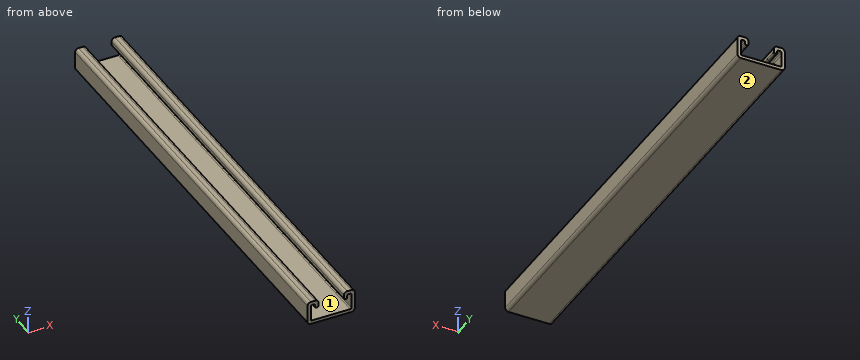
```python
from build123d import *

# Parameters (mm, degrees)
F1_DEPTH = 398
F2_R     = 3
F3_R     = 1


with BuildPart() as f1:
    # F0 (on Front) → F1 (new body)
    with BuildSketch(Plane.XZ):
        Polygon((0, 21), (0, 0), (42, 0), (42, 21), (32.25, 21), (32.25, 14), (35.25, 14), (35.25, 17.75), (39, 17.75), (39, 14), (39, 3), (3, 3), (3, 14), (3.015397, 14), (3.015397, 17.75), (6.765397, 17.75), (6.765397, 14), (9.75, 14), (9.75, 21), align=None)
    extrude(amount=F1_DEPTH)

    # F2
    f2_edges = [f1.edges().sort_by_distance(p)[0] for p in [
        (0, -199, 21),
        (9.75, -199, 21),
        (32.25, -199, 21),
        (42, -199, 21),
        (0, -199, 0),
        (42, -199, 0),
    ]]
    fillet(f2_edges, radius=F2_R)

    # F3
    f3_edges = [f1.edges().sort_by_distance(p)[0] for p in [
        (6.765397, -199, 14),
        (32.25, -199, 14),
        (35.25, -199, 14),
        (9.75, -199, 14),
        (3, -199, 3),
        (39, -199, 3),
        (39, -199, 17.75),
        (3.015397, -199, 17.75),
        (35.25, -199, 17.75),
        (6.765397, -199, 17.75),
    ]]
    fillet(f3_edges, radius=F3_R)


solid = f1.part
```
Input: part model. Units: mm. Frame: model coordinates. Face numbers are marked on the shaded views. A direction names the side the tool comes from. Coordinates: 2 decimals unless noted, no trailing zeros. Loops run counter-clockwise (first coordinate to the right, second up) from the corner with the lowest first, then second, coordinate; pieces in that order, holes last. Notation, with made-up numbers: (43.5, 87.25) -> (75.5, 87.25) arc R23 ccw to (75.5, 120.25) -> close; hole circle Ø2 at (13, 74.25). An arc over 180 degrees is marked (long way). Use a Markdown table: item, result.
1) Material intervals for line 1 along Z through (x, y) = (37, -345); line 2 along X through (y, z) = (-267, 5); line 3 along Z through (x, y) = (6, -281), sorted ascending. Write a range as from..to.
Results found:
| item | result |
|---|---|
| line 1 | z = 0..3, 17.75..21 |
| line 2 | x = 0..3, 39..42 |
| line 3 | z = 0..3, 17.72..21 |
2) Access query for the marked faces 1 and 2. Directions: +Z, -Z, +X, -X, +Y, -Y. A direction counts if a zero-diameter tool reaches every point of the face in a straight line with its end or side. Return the directions, or none.
Results found:
| item | result |
|---|---|
| face 1 | +Y, -Y |
| face 2 | -Z, +X, -X, +Y, -Y |
3) Cut plane C-C (x = 21.5). Return the cut outline in (y, z), then the cut area to 3 significant figures.
Results found:
| item | result |
|---|---|
| outline | (-398, 0) -> (0, 0) -> (0, 3) -> (-398, 3) -> close |
| area | 1,190 mm2 |
4) Cut plane A-A (z = 9). Return the cut outline in (x, y), then the cut area to 3 significant figures.
Results found:
| item | result |
|---|---|
| outline | (0, -398) -> (3, -398) -> (3, 0) -> (0, 0) -> close; (39, -398) -> (42, -398) -> (42, 0) -> (39, 0) -> close |
| area | 2,390 mm2 |
5) Contact query for a flat-ended pin moving along its axis: pin 1 (1.5 mm diameter, centred on x = 29.5, y = -52, fed in from +Z). Output: stop coordinate, or through.
Results found:
| item | result |
|---|---|
| pin 1 | stops at z = 3 |
